```python
from build123d import *

# Parameters (mm, degrees)
BOSS_EXTRUDE1_DEPTH = 3.175
SKETCH2_R           = 1.5875
CUT_EXTRUDE1_DEPTH  = 3.175
BOSS_EXTRUDE2_DEPTH = 3.175
CUT_EXTRUDE2_DEPTH  = 3.175
SKETCH5_W           = 1.5875
SKETCH5_H           = 12.7
CUT_EXTRUDE3_DEPTH  = 10.16
LPATTERN1_COUNT     = 2
LPATTERN1_PITCH     = 25.4
SKETCH8_W           = 38.1
SKETCH8_H           = 46.355
CUT_EXTRUDE6_DEPTH  = 12.7
SKETCH10_R          = 1.5875
CUT_EXTRUDE7_DEPTH  = 7.62
SKETCH11_R          = 6.35
CUT_EXTRUDE8_DEPTH  = 12.7
FILLET1_R           = 25.4
SKETCH13_W          = 25.4
SKETCH13_H          = 177.8
BOSS_EXTRUDE3_DEPTH = 3.175
LPATTERN2_COUNT     = 2
LPATTERN2_PITCH     = 76.2


with BuildPart() as part:
    # Sketch1 → Boss-Extrude1 (new body)
    with BuildSketch(Plane.XY):
        Polygon((0, 0), (-177.8, 0), (-177.8, 349.25), (-25.4, 349.25), align=None)
    extrude(amount=BOSS_EXTRUDE1_DEPTH)

    # Sketch2 → Cut-Extrude1 (cut)
    with BuildSketch(Plane.XY.offset(3.175)):
        with Locations((-127, 133.35)):
            Circle(SKETCH2_R)
        with Locations((-127, 306.07)):
            Circle(SKETCH2_R)
    extrude(amount=-CUT_EXTRUDE1_DEPTH, mode=Mode.SUBTRACT)

    # Sketch3 → Boss-Extrude2 (add)
    with BuildSketch(Plane.XY.offset(3.175)):
        Polygon((-63.5, 88.9), (63.5, 111.29352655), (63.5, 187.49352655), (-63.5, 187.49352655), align=None)
    extrude(amount=-BOSS_EXTRUDE2_DEPTH)

    # Sketch4 → Cut-Extrude2 (cut)
    with BuildSketch(Plane.XY.offset(3.175)):
        Polygon((-44.45, 110.49), (-31.942941537, 112.695331856), (-32.494274501, 115.822096472), (-45.001332964, 113.616764616), align=None)
        Polygon((-6.92882461, 117.105995569), (5.578233853, 119.311327425), (5.026900889, 122.438092041), (-7.480157574, 120.232760185), align=None)
    cut_extrude2 = extrude(amount=-CUT_EXTRUDE2_DEPTH, mode=Mode.SUBTRACT)

    # Sketch5 → Cut-Extrude3 (cut)
    with BuildSketch(Plane.XY.offset(3.175)):
        with Locations((-126.20625, 209.55)):
            Rectangle(SKETCH5_W, SKETCH5_H)
        with Locations((-127.79375, 209.55)):
            Rectangle(SKETCH5_W, SKETCH5_H)
    cut_extrude3 = extrude(amount=-CUT_EXTRUDE3_DEPTH, mode=Mode.SUBTRACT)

    # LPattern1: Cut-Extrude3 ×2
    with Locations(*[(0, i * LPATTERN1_PITCH, 0) for i in range(1, LPATTERN1_COUNT)]):
        add(cut_extrude3, mode=Mode.SUBTRACT)

    # Sketch8 → Cut-Extrude6 (cut)
    with BuildSketch(Plane.XY.offset(3.175)):
        with Locations((-19.05, 23.1775)):
            Rectangle(SKETCH8_W, SKETCH8_H)
    extrude(amount=-CUT_EXTRUDE6_DEPTH, mode=Mode.SUBTRACT)

    # Sketch10 → Cut-Extrude7 (cut)
    with BuildSketch(Plane(origin=(0, 0, 0), x_dir=(-1, 0, 0), z_dir=(0, 0, -1))):
        with Locations((171.45, 20.32)):
            Circle(SKETCH10_R)
        with Locations((44.45, 20.32)):
            Circle(SKETCH10_R)
    extrude(amount=-CUT_EXTRUDE7_DEPTH, mode=Mode.SUBTRACT)

    # Sketch11 → Cut-Extrude8 (cut)
    with BuildSketch(Plane(origin=(0, 0, 0), x_dir=(-1, 0, 0), z_dir=(0, 0, -1))):
        with Locations((156.718, 0)):
            Circle(SKETCH11_R)
        with Locations((65.913, 0)):
            Circle(SKETCH11_R)
    extrude(amount=-CUT_EXTRUDE8_DEPTH, mode=Mode.SUBTRACT)

    # Fillet1
    fillet1_edges = [part.edges().sort_by_distance(p)[0] for p in [
        (-38.1, 46.355, 1.5875),
    ]]
    fillet(fillet1_edges, radius=FILLET1_R)

    # Sketch13 → Boss-Extrude3 (add)
    with BuildSketch(Plane(origin=(0, 0, 0), x_dir=(-1, 0, 0), z_dir=(0, 0, -1))):
        with Locations((12.7, 260.35)):
            Rectangle(SKETCH13_W, SKETCH13_H)
    extrude(amount=-BOSS_EXTRUDE3_DEPTH)

    # LPattern2: Cut-Extrude2 ×2
    with Locations(*[Vector(0.984807753, 0.173648178, 0) * (i * LPATTERN2_PITCH) for i in range(1, LPATTERN2_COUNT)]):
        add(cut_extrude2, mode=Mode.SUBTRACT)


solid = part.part
```
Source: CAD feature listing. Evaluate the final solid. Frame: model axes, mm. Coordinates: 2 decimals unless noted, no trailing zeros. Loops run counter-clockwise (first coordinate to the right, second up) from the corner with the lowest first, then second, coordinate; pieces in that order, holes last. Notation, with made-up numbers: (16.5, -13) - (25.5, -13) arc R27 ccw to (25.5, 20) - close; hole circle Ø4 at (24, 64.25). An arc over 180 degrees is marked (long way). Answer as CSV lines item,"result".
1. Section B-B (z = 0.75). Count the separate pieces of the cut face and the enclosed holes in it, then the cut area to 3 significant figures.
Established:
separate pieces,"1"
enclosed holes,"9"
area,"65,000 mm2"
2. Contact query for flat-ended pins moving along their axis: pin 1 (10 mm diameter, centred on x = -24.5, y = 269.5, fed in from -Z); pin 2 (1.9 mm diameter, centred on x = -44.45, y = 20.32, fed in from +Z); pin 3 (1 mm diameter, centred on x = -7.5, z = 1, fed in from -Y) (3 decimals); pin 4 (1 mm diameter, centred on x = 21, z = 1, fed in from +Y). Output: stop coordinate, or through.
Established:
pin 1,"stops at z = 0"
pin 2,"passes through"
pin 3,"stops at y = 46.355"
pin 4,"stops at y = 187.49"
3. Ray query, line 1 (Y direction, x = -127, z = 0.95); line 2 (X direction, y = 306.07, z = 1); line 3 (Y direction, x = -171.45, z = 1.65). Return the intervals inside material, ascending.
Established:
line 1,"y = 0 to 131.76, 134.94 to 203.2, 215.9 to 228.6, 241.3 to 304.48, 307.66 to 349.25"
line 2,"x = -177.8 to -128.59, -125.41 to 0"
line 3,"y = 0 to 18.73, 21.91 to 349.25"
4. Section A-A (y = 234). Return loops of the section in (x, z) (1 decimal), then the cut area to 3 significant figures.
Established:
outline,"(-177.8, 0) - (-128.6, 0) - (-128.6, 3.2) - (-177.8, 3.2) - close; (-125.4, 0) - (0, 0) - (0, 3.2) - (-125.4, 3.2) - close"
area,"554 mm2"
5. Section D-D (x = 16.5). Return loops of the section in (y, z) (3 decimals), then the cut area to 3 significant figures.
Established:
outline,"(103.006, 0) - (187.494, 0) - (187.494, 3.175) - (103.006, 3.175) - close"
area,"268 mm2"
6. Section C-C (y = 55). Return loops of the section in (x, z) (3 decimals), then the cut area to 3 significant figures.
Established:
outline,"(-177.8, 0) - (-4, 0) - (-4, 3.175) - (-177.8, 3.175) - close"
area,"552 mm2"
7. Mould query, pull axis Z, two halves, no side actions, for faces 1 (the flat face through (-82, 177, 0)), 2 (the flat face through (27.661, 104.974, 1.61)), 3 (the flat face through (-82, 177, 3.175)). Classes: released by +Z, released by -Z, zero draft, split by the parting line, or undercut.
Established:
face 1,"released by -Z"
face 2,"zero draft"
face 3,"released by +Z"
